Autodesk Inventor part; units mm, degrees
ref_plane "YZ Plane" through (0, 0, 0) normal (1, 0, 0) x (0, 1, 0)
ref_plane "XZ Plane" through (0, 0, 0) normal (0, 1, 0) x (-1, 0, 0)
ref_plane "XY Plane" through (0, 0, 0) normal (0, 0, 1) x (1, 0, 0)
sketch "Sketch1" plane through (0, 0, 0) normal (0, 1, 0) x (-1, 0, 0)
  arc A0 (-31.588, -3.2035) -> (31.588, 3.2035) centre (0, 0) ccw
  line L0 (0, 0) -> (-31.588, -3.2035) construction
  line L1 (0, 0) -> (31.588, 3.2035) construction
  line L2 (31.588, 3.2035) -> (-31.588, -3.2035)
revolve "Revolution1" add sketch "Sketch1" angle 180 about axis through (0, 0, 0) along (0.9948968, 0, -0.1008975)
sketch "Sketch2" plane through (0, 0, 0) normal (0, -1, 0) x (1, 0, 0)
  circle A0 centre (0, 0) radius 31.75
extrude "Extrusion1" cut sketch "Sketch2" against normal blind 30.48 keep common part
sketch "Sketch3" plane through (0, 0, 0) normal (0, -1, 0) x (1, 0, 0)
  line L0 (0, 0) -> (0, -27.94)
  circle A0 centre (0, 0) radius 8.89
  line L1 (0, 0) -> (0, 25.4)
  circle A1 centre (0, 0) radius 27.94
  circle A2 centre (0, 0) radius 25.4
  dimension "d7" = 27.94
  dimension "d8" = 25.4
extrude "Extrusion2" cut sketch "Sketch3" against normal blind 3.175
sketch "Sketch4" plane through (0, 30.48, 0) normal (0, 1, 0) x (1, 0, 0)
  circle A0 centre (0, 0) radius 1.5875
  dimension "d11" = 3.175
extrude "Extrusion3" cut sketch "Sketch4" against normal blind 6.35
sketch "Sketch5" plane through (0, 0, 0) normal (0, -1, 0) x (1, 0, 0)
  circle A0 centre (0, 0) radius 1.5875
  circle A1 centre (0, 0) radius 31.75
  circle A2 centre (0, 0) radius 27.94
extrude "Extrusion4" cut sketch "Sketch5" against normal blind 3.175 contours A1
properties part number "ball tops"
Input: part model. Units: mm. Frame: model coordinates. A direction names the side the tool comes from. Coordinates: 2 decimals unless noted, no trailing zeros. Write each loop counter-clockwise with the first axis right and the second up, starting at its lowest first coordinate (ties: lowest second). Pieces come first, ordered by that corner, then holes. Notation, with made-up numbers: M 26.25,2.5 L 51.25,2.5 A16 ccw 51.25,28.5 Z; hole C 85,67 d4. An arc over 180 degrees is marked long. Use one line per item in the form item = value.
Q1. Section B-B (z = 0). Return loops of the section in (x, y) (1 decimal), plus the area to 3 significant figures.
Answer below:
outline = M -31.6,3.2 L -25.4,3.2 L -25.4,0 L 25.4,0 L 25.4,3.2 L 31.6,3.2 A31.8 ccw 8.9,30.5 L 1.6,30.5 L 1.6,24.1 L -1.6,24.1 L -1.6,30.5 L -8.9,30.5 A31.8 ccw Z
area = 1,510 mm²
Q2. Section A-A (x = 0). Return loops of the section in (y, z) (1 decimal).
Answer below:
outline = M 0,-25.4 L 3.2,-25.4 L 3.2,-31.6 A31.8 ccw 30.5,-8.9 L 30.5,-1.6 L 24.1,-1.6 L 24.1,1.6 L 30.5,1.6 L 30.5,8.9 A31.8 ccw 3.2,31.6 L 3.2,25.4 L 0,25.4 Z
Q3. Section D-D (z = -15). Return loops of the section in (x, y) (3 decimals), plus the area to 3 significant figures.
Answer below:
outline = M -27.803,3.175 L -20.498,3.175 L -20.498,0 L 20.498,0 L 20.498,3.175 L 27.803,3.175 A27.983 ccw Z
area = 1,180 mm²
Q4. Set-up query: faces 1 (the face through (0, 0, 0)), 2 (the face through (-5.506, 1.565, -24.796)), 3 (the face through (-0.34, 27.35, 1.55)). Return all of +Z, -Z, +X, -X, +Y, -Y with unobstructed straight access to the full face (end or side cutting, diameter ignored); none if empty.
Answer below:
face_1 = +Z, -Z, +X, -X, -Y
face_2 = -Y
face_3 = +Y
Q5. First-contact query: pin 1 (6 mm diameter, centred on x = -6, y = 15.5, fed in from -Z); pin 2 (5 mm diameter, centred on y = 6.5, z = -1.5, fed in from -X); pin 3 (3 mm diameter, centred on y = 15, z = 0.5, fed in from -X). Flat tips, straight axial feed; report the tip coordinate or a pass-through.
Answer below:
pin_1 = -28.68
pin_2 = -31.47
pin_3 = -28.73
Q6. Draft query along X for faces 4 (the face through (0, 24.13, 0)), 5 (the face through (0, 30.48, -2)). Return one class per face: released by +X, released by -X, zero draft, split by the parting line, or undercut.
Answer below:
face_4 = undercut
face_5 = zero draft
Q7. Section C-C (y = 13). Return loops of the section in (x, z).
Answer below:
outline = C 0,0 d57.93
Q8. Material intervals for probe 1 along Z at (x, y) = (0, 28.75); probe 2 along X at (y, z) = (27.5, 0); probe 3 along X at (y, z) = (28.5, 0), sorted ascending. Write a range as from..to.
Answer below:
probe_1 = -13.47..-1.59, 1.59..13.47
probe_2 = -15.87..-1.59, 1.59..15.87
probe_3 = -13.99..-1.59, 1.59..13.99
